Input: part model. Units: mm. Frame: model coordinates. Face numbers are marked on the shaded views. A direction names the side the tool comes from. Give positions to 0.01 mm unless a question says otherwise; leave off trailing zeros. Order: outer loops, then holes, each group sorted by start corner. A loop starts at its lowest first (then second) coordinate and runs counter-clockwise, first axis right, second up. Notation, with made-up numbers: M 4.5,31.5 L 45.5,31.5 A17 cw 45.5,63.5 Z; hole C 10,2.25 d11. An arc over 180 degrees is marked long. Use a Markdown table: item, result.
from build123d import *

# Parameters (mm, degrees)
SKETCH_W            = 47.7
SKETCH_H            = 23.7
PAD_DEPTH           = 14.4
SKETCH001_R         = 3.6
PAD001_DEPTH        = 2.7
LINEARPATTERN_COUNT = 4
LINEARPATTERN_PITCH = 11.9
SKETCH002_W         = 44.1
SKETCH002_H         = 20.1
SKETCH002_R         = 4.8825
SKETCH002_R_2       = 3.6
POCKET_DEPTH        = 12


with BuildPart() as part:
    # Sketch → Pad (new body)
    with BuildSketch(Plane.XY):
        Rectangle(SKETCH_W, SKETCH_H)
    extrude(amount=PAD_DEPTH)

    # Sketch001 (on Face6 of Pad) → Pad001 (join)
    with BuildSketch(Plane.XY.offset(14.4)):
        with Locations((-17.85, -5.85)):
            Circle(SKETCH001_R)
        with Locations((-17.85, 5.85)):
            Circle(SKETCH001_R)
    pad001 = extrude(amount=PAD001_DEPTH)

    # LinearPattern: Pad001 ×4
    with Locations(*[(i * LINEARPATTERN_PITCH, 0, 0) for i in range(1, LINEARPATTERN_COUNT)]):
        add(pad001)

    # Sketch002 (on Face4 of LinearPattern) → Pocket (cut)
    with BuildSketch(Plane(origin=(0, 0, 0), x_dir=(1, 0, 0), z_dir=(0, 0, -1))):
        Rectangle(SKETCH002_W, SKETCH002_H)
        with Locations((-11.85, 0)):
            Circle(SKETCH002_R, mode=Mode.SUBTRACT)
        with Locations((0.15, 0)):
            Circle(SKETCH002_R, mode=Mode.SUBTRACT)
        with Locations((12.15, 0)):
            Circle(SKETCH002_R, mode=Mode.SUBTRACT)
        with Locations((-11.85, 0)):
            Circle(SKETCH002_R_2)
        with Locations((0.15, 0)):
            Circle(SKETCH002_R_2)
        with Locations((12.15, 0)):
            Circle(SKETCH002_R_2)
    extrude(amount=-POCKET_DEPTH, mode=Mode.SUBTRACT)


solid = part.part
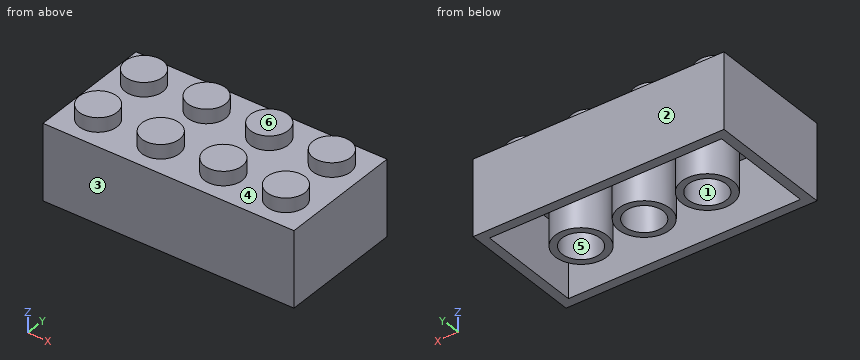
1) Material intervals for line 1 (Y direction, x = 0.15, z = 4.25); line 2 (Y direction, x = -14.5, z = 10.25); line 3 (X direction, y = -7.5, z = 8.75), sorted ascending. Write a range as from..to.
Response values:
| item | result |
|---|---|
| line 1 | y = -11.85..-10.05, -4.88..-3.6, 3.6..4.88, 10.05..11.85 |
| line 2 | y = -11.85..-10.05, -4.1..-2.44, 2.44..4.1, 10.05..11.85 |
| line 3 | x = -23.85..-22.05, 22.05..23.85 |
2) Reachability of the marked faces 4, 5 and 6 from +Z, -Z, +X, -X, +Y, -Y: full face, straight path, thin tool, end or side. Return the list, or none.
Response values:
| item | result |
|---|---|
| face 4 | +Z |
| face 5 | -Z |
| face 6 | +Z, +X, -X, +Y, -Y |
3) Cut plane A-A on z = 15.75. Return loops of the section in (x, y), and give its area (3 significant figures).
Response values:
| item | result |
|---|---|
| outline | C -17.85,-5.85 d7.2; C -17.85,5.85 d7.2; C -5.95,-5.85 d7.2; C -5.95,5.85 d7.2; C 5.95,-5.85 d7.2; C 5.95,5.85 d7.2; C 17.85,-5.85 d7.2; C 17.85,5.85 d7.2 |
| area | 326 mm² |
4) Cut plane D-D on x = 0.15. Return loops of the section in (y, z), and give its area (3 significant figures).
Response values:
| item | result |
|---|---|
| outline | M -11.85,0 L -10.05,0 L -10.05,12 L -4.88,12 L -4.88,0 L -3.6,0 L -3.6,12 L 3.6,12 L 3.6,0 L 4.88,0 L 4.88,12 L 10.05,12 L 10.05,0 L 11.85,0 L 11.85,14.4 L -11.85,14.4 Z |
| area | 131 mm² |
5) Mould query, pull axis Y, two halves, no side actions, for the marked faces 1, 2 and 3. Classes: released by +Y, released by -Y, zero draft, split by the parting line, or undercut.
Response values:
| item | result |
|---|---|
| face 1 | undercut |
| face 2 | released by +Y |
| face 3 | released by -Y |
6) First-contact query: pin 1 Ø6 at (x, y) = (12.15, 0) entering from +Z; pin 2 Ø6.5 at (x, y) = (-11.85, 0) entering from -Z. Flat tips, straight axial feed; report the tip coordinate or a pass-through.
Response values:
| item | result |
|---|---|
| pin 1 | stops at z = 14.4 |
| pin 2 | stops at z = 12 |
7) Cut plane B-B on z = 10. State how many separate pieces and enclosed holes the cut face has, and give its area (3 significant figures).
Response values:
| item | result |
|---|---|
| separate pieces | 4 |
| enclosed holes | 4 |
| area | 347 mm² |
8) Cut plane C-C on y = 5.85. Return loops of the section in (x, z), and give its area (3 significant figures).
Response values:
| item | result |
|---|---|
| outline | M -23.85,0 L -22.05,0 L -22.05,12 L 22.05,12 L 22.05,0 L 23.85,0 L 23.85,14.4 L 21.45,14.4 L 21.45,17.1 L 14.25,17.1 L 14.25,14.4 L 9.55,14.4 L 9.55,17.1 L 2.35,17.1 L 2.35,14.4 L -2.35,14.4 L -2.35,17.1 L -9.55,17.1 L -9.55,14.4 L -14.25,14.4 L -14.25,17.1 L -21.45,17.1 L -21.45,14.4 L -23.85,14.4 Z |
| area | 235 mm² |
